Source: CAD feature listing. Evaluate the final solid. Frame: model axes, mm. A direction names the side the tool comes from. Give positions to 0.01 mm unless a question says otherwise; leave off trailing zeros. Loops run counter-clockwise (first coordinate to the right, second up) from the corner with the lowest first, then second, coordinate; pieces in that order, holes last. Notation, with made-up numbers: (69, 17.5) -> (92, 17.5) arc R5 cw to (92, 26.5) -> close; hole circle Ø10 at (89, 36). An arc over 180 degrees is marked (long way). Answer as a JSON object with one key per item and string values. Group by question number.
from build123d import *

# Parameters (mm, degrees)
SOCKET_1_SKETCH_W = 16.2
SOCKET_1_SKETCH_H = 3.175
SOCKET_2_SKETCH_W = 16.2
SOCKET_2_SKETCH_H = 3.175


with BuildPart() as part:
    # Union_T4 Sketch → Union_T4 (revolve)
    with BuildSketch(Plane.XY, mode=Mode.PRIVATE) as union_t4_sk:
        Polygon((-20.45, 0), (-20.45, 7.722), (-3.45, 7.722), (3.45, 7.722), (20.45, 7.722), (20.45, 0), align=None)
    revolve(union_t4_sk.sketch.rotate(Axis((-1000, 0, 0), (1, 0, 0)), 90), axis=Axis((-1000, 0, 0), (1, 0, 0)))

    # Socket 1 Sketch → Socket 1 (revolve, cut)
    with BuildSketch(Plane.XY, mode=Mode.PRIVATE) as socket_1_sk:
        with Locations((-13.35, 1.5875)):
            Rectangle(SOCKET_1_SKETCH_W, SOCKET_1_SKETCH_H)
    revolve(socket_1_sk.sketch.rotate(Axis((-1000, 0, 0), (1, 0, 0)), 90), axis=Axis((-1000, 0, 0), (1, 0, 0)), mode=Mode.SUBTRACT)

    # Socket 2 Sketch → Socket 2 (revolve, cut)
    with BuildSketch(Plane.XY, mode=Mode.PRIVATE) as socket_2_sk:
        with Locations((13.35, 1.5875)):
            Rectangle(SOCKET_2_SKETCH_W, SOCKET_2_SKETCH_H)
    revolve(socket_2_sk.sketch.rotate(Axis((-1000, 0, 0), (1, 0, 0)), 90), axis=Axis((-1000, 0, 0), (1, 0, 0)), mode=Mode.SUBTRACT)


solid = part.part
(1) Access query for faces 1 (the face through (-12.74, 1.93, -2.52)), 2 (the face through (5.25, 0, 0)), 3 (the face through (-20.45, -0.108, -3.324)). Directions: +Z, -Z, +X, -X, +Y, -Y. A direction counts if a zero-diameter tool reaches every point of the face in a straight line with its end or side. Return the directions, or none.
(2) Section query D-D on y = -4. Return the cut outline in (x, z), plus the area to 3 significant figures.
(3) Section query A-A on z = 0. Return the cut outline in (x, y) (3 decimals).
(4) Mould query, pull axis Y, two halves, no side actions, for faces 4 (the face through (20.45, -0.108, 3.324)), 5 (the face through (-0.286, -7.656, -1.005)), 6 (the face through (-5.25, 0, 0)). Classes: pulls with the +Y half, pulls with the -Y half, needs draft (parallel to the pull), parting line crosses it, or undercut.
(5) First-contact query: pin 1 (2 mm diameter, centred on x = 7.5, y = -3, fed in from +Z); pin 2 (4 mm diameter, centred on y = 0, z = 0, fed in from +X); pin 3 (2 mm diameter, centred on x = -5, z = -3.5, fed in from +Y). Flat tips, straight axial feed; report the tip coordinate or a pass-through.
(6) Material intervals for line 1 (Y direction, x = -8.75, z = 0) (3 decimals); line 2 (X direction, y = 1.25, z = 0.75); line 3 (Z direction, x = -5.5, y = 0.5), sorted ascending. Write a range as from..to.
(7) Section query B-B on x = -16.5. Return the cut outline in (y, z) (3 decimals), plus the area to 3 significant figures.
Result:
{
 "1": {"face 1": "-X", "face 2": "+X", "face 3": "+Z, -Z, -X, +Y, -Y"},
 "2": {"outline": "(-20.45, -6.61) -> (20.45, -6.61) -> (20.45, 6.61) -> (-20.45, 6.61) -> close", "area": "540 mm²"},
 "3": {"outline": "(-20.45, -7.722) -> (20.45, -7.722) -> (20.45, -3.175) -> (5.25, -3.175) -> (5.25, 3.175) -> (20.45, 3.175) -> (20.45, 7.722) -> (-20.45, 7.722) -> (-20.45, 3.175) -> (-5.25, 3.175) -> (-5.25, -3.175) -> (-20.45, -3.175) -> close"},
 "4": {"face 4": "needs draft", "face 5": "parting line crosses it", "face 6": "undercut"},
 "5": {"pin 1": "z = 7.46", "pin 2": "x = 5.25", "pin 3": "y = 7.31"},
 "6": {"line 1": "-7.722..-3.175, 3.175..7.722", "line 2": "-5.25..5.25", "line 3": "-7.71..-3.14, 3.14..7.71"},
 "7": {"outline": "circle Ø15.444 at (0, 0); hole circle Ø6.35 at (0, 0)", "area": "156 mm²"}
}
